Build history of the part. All positions in model axes, mm. Face numbers are marked on the shaded views. A direction names the side the tool comes from. Round coordinates to 2 decimals unless told otherwise and drop trailing zeros. Loops run counter-clockwise (first coordinate to the right, second up) from the corner with the lowest first, then second, coordinate; pieces in that order, holes last. Notation, with made-up numbers: (83.25, 17.5) - (114.25, 17.5) arc R38 cw to (114.25, 56.5) - close; hole circle Ø10 at (5.25, 42.5). An arc over 180 degrees is marked (long way). Answer as CSV lines item,"result". Start each with the question number.
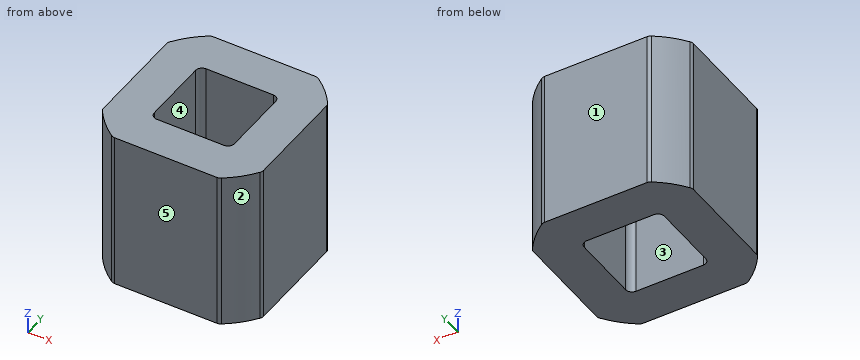
Autodesk Inventor part; units mm, degrees
ref_plane "YZ Plane" through (0, 0, 0) normal (1, 0, 0) x (0, 1, 0)
ref_plane "XZ Plane" through (0, 0, 0) normal (0, 1, 0) x (-1, 0, 0)
ref_plane "XY Plane" through (0, 0, 0) normal (0, 0, 1) x (1, 0, 0)
sketch "Sketch1" plane through (0, 0, 0) normal (0, 0, 1) x (1, 0, 0)
  line L0 (-3.175, -3.175) -> (3.175, -3.175)
  line L1 (3.175, -3.175) -> (3.175, 3.175)
  line L2 (3.175, 3.175) -> (-3.175, 3.175)
  line L3 (-3.175, 3.175) -> (-3.175, -3.175)
  line L4 (-3.175, -3.175) -> (3.175, 3.175) construction
  line L5 (3.175, -3.175) -> (-3.175, 3.175) construction
  circle A0 centre (0, 0) radius 3.81
  point P0 (2.1061, -3.175)
  point P1 (3.175, -2.1061)
  point P2 (3.175, 2.1061)
  point P3 (2.1061, 3.175)
  point P4 (-2.1061, 3.175)
  point P5 (-3.175, 2.1061)
  point P6 (-3.175, -2.1061)
  point P7 (-2.1061, -3.175)
  dimension "d0" = 7.62
  dimension "d1" = 6.35
extrude "Extrusion1" add sketch "Sketch1" against normal blind 12.7 contours A0 L3 L2 L1 L0
sketch "Sketch2" plane through (0, 0, 0) normal (0, 0, 1) x (1, 0, 0)
  arc A0 (-3.175, -2.1061) -> (-2.1061, -3.175) centre (0, 0) ccw construction
  line L0 (-1.5875, -1.5875) -> (1.5875, -1.5875)
  line L1 (1.5875, -1.5875) -> (1.5875, 1.5875)
  line L2 (1.5875, 1.5875) -> (-1.5875, 1.5875)
  line L3 (-1.5875, 1.5875) -> (-1.5875, -1.5875)
  line L4 (-1.5875, -1.5875) -> (1.5875, 1.5875) construction
  line L5 (1.5875, -1.5875) -> (-1.5875, 1.5875) construction
  dimension "d7" = 3.175
extrude "Extrusion2" cut sketch "Sketch2" against normal blind 12.7
fillet "Fillet1" radius 0.254 12 edges at (-1.5875, -1.5875, -6.35) (-1.5875, 1.5875, -6.35) (1.5875, 1.5875, -6.35) (1.5875, -1.5875, -6.35) (2.1061, 3.175, -6.35) (3.175, 2.1061, -6.35) (3.175, -2.1061, -6.35) (2.1061, -3.175, -6.35) (-2.1061, -3.175, -6.35) (-3.175, -2.1061, -6.35) (-3.175, 2.1061, -6.35) (-2.1061, 3.175, -6.35)
sketch "Sketch3" plane through (0, 0, 0) normal (0, 0, 1) x (1, 0, 0)
  line L0 (-7.3828, 5.7639) -> (4.9041, 5.7639)
  line L1 (4.9041, 5.7639) -> (4.9041, -5.3132)
  line L2 (4.9041, -5.3132) -> (-7.3828, -5.3132)
  line L3 (-7.3828, -5.3132) -> (-7.3828, 5.7639)
  point P0 (0, 0)
extrude "Extrusion3" cut sketch "Sketch3" against normal blind 6.35
properties part number "HS Shaft Adapter Square"
Q1. Wall check: probe 1 along X at (y, z) = (1, -10.5) (1 decimal); probe 2 along Y at (x, z) = (-1.5, -7.75) (3 decimals). Give the ranges that are in metal, low to high. Write a range as [from, to].
Q2. Band-saw the part on D-D, the plane x = 2.5. List the corners of the cut face in (y, z).
Q3. Two-plate mould, pull along X, no slides. Class the marked faces 1, 2 and 3: released by +X, released by -X, zero draft, split by the parting line, or undercut.
Q4. Tool access for the marked faces 4 and 5: list every direction of +Z, -Z, +X, -X, +Y, -Y with a clear straight run to the whole face (end or side of a thin tool).
Reported:
1,probe 1,"x = [-3.2, -1.6], [1.6, 3.2]"
1,probe 2,"y = [-3.175, -1.525], [1.525, 3.175]"
2,outline,"(-2.88, -12.7) - (2.88, -12.7) - (2.88, -6.35) - (-2.88, -6.35) - close"
3,face 1,"zero draft"
3,face 2,"released by +X"
3,face 3,"undercut"
4,face 4,"+Z, -Z"
4,face 5,"+Z, -Z, +X, -X, -Y"
